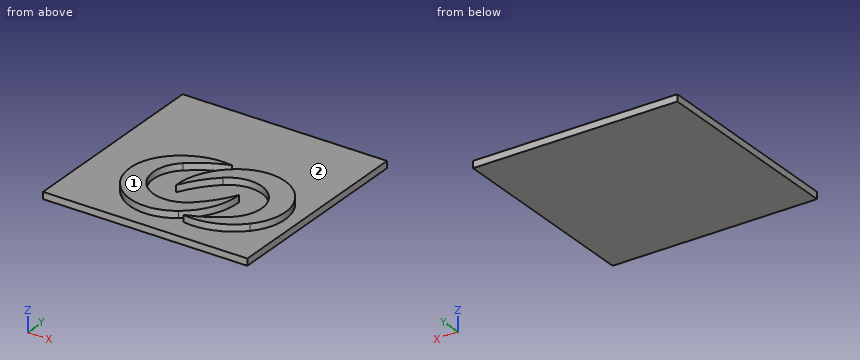
from build123d import *

# Parameters (mm, degrees)
SKICA1_W                = 300
SKICA1_H                = 300
P_IDAT_VYSUNUT_M1_DEPTH = 10
P_IDAT_VYSUNUT_M3_DEPTH = 10


with BuildPart() as part:
    # Skica1 → Přidat vysunutím1 (new body)
    with BuildSketch(Plane.XY):
        with Locations((150, 150)):
            Rectangle(SKICA1_W, SKICA1_H)
    extrude(amount=P_IDAT_VYSUNUT_M1_DEPTH)

    # Skica3 → Přidat vysunutím3 (add)
    with BuildSketch(Plane.XY.offset(10)):
        with BuildLine():
            ThreePointArc((161.258214426, 169.732529164), (118.091173044, 166.070333412), (81.747818606, 142.491407915))
            ThreePointArc((81.747818606, 142.491407915), (80.157704047, 48.826419384), (173.139331363, 37.421353736))
            ThreePointArc((173.139331363, 37.421353736), (201.527121298, 70.146550787), (211.135953458, 112.38960328))
            ThreePointArc((211.135953458, 112.38960328), (195.41469161, 86.876535147), (174.935524438, 64.997814169))
            ThreePointArc((174.935524438, 64.997814169), (104.302093893, 69.827572661), (109.307122532, 140.448800107))
            ThreePointArc((109.307122532, 140.448800107), (133.812696433, 157.698483219), (161.258214426, 169.732529164))
        make_face()
        with BuildLine():
            ThreePointArc((263.117659489, 59.733740684), (226.718588511, 36.240916857), (183.542998572, 32.680920678))
            ThreePointArc((183.542998572, 32.680920678), (211.01692785, 44.649961145), (235.56326825, 61.841583891))
            ThreePointArc((235.56326825, 61.841583891), (240.735464455, 132.450765052), (170.113665313, 137.447720489))
            ThreePointArc((170.113665313, 137.447720489), (149.582762041, 115.617541137), (133.801147174, 90.141761426))
            ThreePointArc((133.801147174, 90.141761426), (143.509954364, 132.361948569), (171.975135093, 165.019851524))
            ThreePointArc((171.975135093, 165.019851524), (264.929502664, 153.394702482), (263.117659489, 59.733740684))
        make_face()
    extrude(amount=P_IDAT_VYSUNUT_M3_DEPTH)


solid = part.part
Source: CAD feature listing. Evaluate the final solid. Frame: model axes, mm. Face numbers are marked on the shaded views. Round coordinates to 2 decimals unless told otherwise and drop trailing zeros. Loops run counter-clockwise (first coordinate to the right, second up) from the corner with the lowest first, then second, coordinate; pieces in that order, holes last. Notation, with made-up numbers: (88, 39) - (146, 39) arc R27 cw to (146, 76) - close; hole circle Ø7 at (-33, 34.25). An arc over 180 degrees is marked (long way). Write item = value, one per line. Start each with the question number.
Item 1: Material intervals for line 1 (X direction, y = 68, z = 12); line 2 (Z direction, x = 111.5, y = 186.5); line 3 (X direction, y = 77, z = 16), sorted ascending.
Item 2: Section query C-C on y = 98.5. Output: boundary loops of the cut face in (x, z).
Item 3: Mould query, pull axis Y, two halves, no side actions, for the marked faces 1 and 2. Classes: released by +Y, released by -Y, zero draft, split by the parting line, or undercut.
Item 4: Section query B-B on x = 125. Output: boundary loops of the cut face in (y, z), plus the area to 3 significant figures.
Item 5: First-contact query: pin 1 Ø1 at (x, y) = (212, 212) entering from -Z; pin 2 Ø4 at (x, z) = (99.5, 17) entering from +Y. Flat tips, straight axial feed; report the tip coordinate or a pass-through.
Item 6: Section query A-A on z = 16. Output: boundary loops of the cut face in (x, y).
Item 7: Section query D-D on x = 220.5. Output: boundary loops of the cut face in (y, z), plus the area to 3 significant figures.
Results list:
q1.line_1 = 68.29 to 105.97, 178.27 to 200.4, 241.58 to 269.75
q1.line_2 = 0 to 10
q1.line_3 = 65.26 to 99.1, 187.18 to 204.64, 247.47 to 274.98
q2.outline = (0, 0) - (300, 0) - (300, 10) - (281.42, 10) - (281.42, 20) - (252.92, 20) - (252.92, 10) - (210.35, 10) - (210.35, 20) - (203.46, 20) - (203.46, 10) - (138.22, 10) - (138.22, 20) - (134.03, 20) - (134.03, 10) - (92.2, 10) - (92.2, 20) - (63.07, 20) - (63.07, 10) - (0, 10) - close
q3.face_1 = zero draft
q3.face_2 = undercut
q4.outline = (0, 0) - (300, 0) - (300, 10) - (168.13, 10) - (168.13, 20) - (152.32, 20) - (152.32, 10) - (55.63, 10) - (55.63, 20) - (25.22, 20) - (25.22, 10) - (0, 10) - close
q4.area = 3,460 mm²
q5.pin_1 = 0
q5.pin_2 = 158.41
q6.outline = (81.75, 142.49) arc R70.01 ccw to (173.14, 37.42) arc R89.15 ccw to (211.14, 112.39) arc R150 cw to (174.94, 65) arc R50 cw to (109.31, 140.45) arc R150 cw to (161.26, 169.73) arc R89.15 ccw to start; (133.8, 90.14) arc R150 cw to (170.11, 137.45) arc R50 cw to (235.56, 61.84) arc R150 cw to (183.54, 32.68) arc R89.15 ccw to (263.12, 59.73) arc R70.01 ccw to (171.98, 165.02) arc R89.15 ccw to start
q7.outline = (0, 0) - (300, 0) - (300, 10) - (177.07, 10) - (177.07, 20) - (146.54, 20) - (146.54, 10) - (50.44, 10) - (50.44, 20) - (34.38, 20) - (34.38, 10) - (0, 10) - close
q7.area = 3,470 mm²
